Autodesk Inventor part; units mm, degrees
ref_plane "YZ Plane" through (0, 0, 0) normal (1, 0, 0) x (0, 1, 0)
ref_plane "XZ Plane" through (0, 0, 0) normal (0, 1, 0) x (-1, 0, 0)
ref_plane "XY Plane" through (0, 0, 0) normal (0, 0, 1) x (1, 0, 0)
sketch "Эскиз1" plane through (0, 0, 0) normal (0, 1, 0) x (-1, 0, 0)
  arc A0 (13.2517, 5.1196) -> (11.6396, 8.8847) centre (11.8859, 6.7625) ccw
  line L0 (11.6396, 8.8847) -> (3.5765, 5.9707)
  line L1 (3.5765, 5.9707) -> (2.1921, 14.0362)
  arc A1 (2.1921, 14.0362) -> (-1.8746, 14.5225) centre (0.0865, 13.6747) ccw
  line L2 (-1.8746, 14.5225) -> (-3.3825, 6.0827)
  line L3 (-3.3825, 6.0827) -> (-11.0596, 8.9165)
  arc A2 (-11.0596, 8.9165) -> (-13.5142, 5.6378) centre (-11.7994, 6.9122) ccw
  line L4 (-13.5142, 5.6378) -> (-6.959, 0.112)
  line L5 (-6.959, 0.112) -> (-13.2517, -5.1196)
  arc A3 (-13.2517, -5.1196) -> (-11.6396, -8.8847) centre (-11.8859, -6.7625) ccw
  line L6 (-11.6396, -8.8847) -> (-3.5765, -5.9707)
  line L7 (-3.5765, -5.9707) -> (-2.1921, -14.0362)
  arc A4 (-2.1921, -14.0362) -> (1.8746, -14.5225) centre (-0.0865, -13.6747) ccw
  line L8 (1.8746, -14.5225) -> (3.3825, -6.0827)
  line L9 (3.3825, -6.0827) -> (11.0596, -8.9165)
  arc A5 (11.0596, -8.9165) -> (13.5142, -5.6378) centre (11.7994, -6.9122) ccw
  line L10 (13.5142, -5.6378) -> (6.959, -0.112)
  line L11 (6.959, -0.112) -> (13.2517, 5.1196)
  circle A6 centre (6.6709, 3.7954) radius 1
  circle A7 centre (11.8859, 6.7625) radius 1
  circle A8 centre (9.2109, -5.3958) radius 1
  circle A9 centre (-0.0485, -7.6748) radius 1
  circle A10 centre (-0.0865, -13.6747) radius 1
  circle A11 centre (-9.2784, -5.2789) radius 1
  circle A12 centre (-6.6223, 3.8794) radius 1
  circle A13 centre (-11.7994, 6.9122) radius 1
  circle A14 centre (0.0675, 10.6748) radius 1
  circle A15 centre (0, 0) radius 4.75
  circle A16 centre (0.0865, 13.6747) radius 1
  circle A17 centre (0.0485, 7.6748) radius 1
  circle A18 centre (-9.2109, 5.3958) radius 1
  circle A19 centre (-11.8859, -6.7625) radius 1
  circle A20 centre (-6.6709, -3.7954) radius 1
  circle A21 centre (-0.0675, -10.6748) radius 1
  circle A22 centre (11.7994, -6.9122) radius 1
  circle A23 centre (6.6223, -3.8794) radius 1
  circle A24 centre (9.2784, 5.2789) radius 1
  circle A25 centre (0, 0) radius 1.875
  circle A26 centre (0, 0) radius 20
  circle A27 centre (0, 0) radius 17.5
  point P0 (0, 0)
  dimension "d0" = 40
  dimension "d1" = 35
extrude "Выдавливание1" add sketch "Эскиз1" along normal blind 2 contours L11 L10 A5 L9 L8 A4 L7 L6 A3 L5 L4 A2 L3 L2 A1 L1 L0 A0 | A26 | A27
sketch "Эскиз2" plane through (0, 2, 0) normal (0, 1, 0) x (1, 0, 0)
  arc A0 (13.2517, 5.1196) -> (11.6396, 8.8847) centre (11.8859, 6.7625) ccw
  line L0 (11.6396, 8.8847) -> (3.5765, 5.9707)
  line L1 (3.5765, 5.9707) -> (2.1921, 14.0362)
  arc A1 (2.1921, 14.0362) -> (-1.8746, 14.5225) centre (0.0865, 13.6747) ccw
  line L2 (-1.8746, 14.5225) -> (-3.3825, 6.0827)
  line L3 (-3.3825, 6.0827) -> (-11.0596, 8.9165)
  arc A2 (-11.0596, 8.9165) -> (-13.5142, 5.6378) centre (-11.7994, 6.9122) ccw
  line L4 (-13.5142, 5.6378) -> (-6.959, 0.112)
  line L5 (-6.959, 0.112) -> (-13.2517, -5.1196)
  arc A3 (-13.2517, -5.1196) -> (-11.6396, -8.8847) centre (-11.8859, -6.7625) ccw
  line L6 (-11.6396, -8.8847) -> (-3.5765, -5.9707)
  line L7 (-3.5765, -5.9707) -> (-2.1921, -14.0362)
  arc A4 (-2.1921, -14.0362) -> (1.8746, -14.5225) centre (-0.0865, -13.6747) ccw
  line L8 (1.8746, -14.5225) -> (3.3825, -6.0827)
  line L9 (3.3825, -6.0827) -> (11.0596, -8.9165)
  arc A5 (11.0596, -8.9165) -> (13.5142, -5.6378) centre (11.7994, -6.9122) ccw
  line L10 (13.5142, -5.6378) -> (6.959, -0.112)
  line L11 (6.959, -0.112) -> (13.2517, 5.1196)
  circle A6 centre (6.6709, 3.7954) radius 1
  circle A7 centre (11.8859, 6.7625) radius 1
  circle A8 centre (9.2109, -5.3958) radius 1
  circle A9 centre (-0.0485, -7.6748) radius 1
  circle A10 centre (-0.0865, -13.6747) radius 1
  circle A11 centre (-9.2784, -5.2789) radius 1
  circle A12 centre (-6.6223, 3.8794) radius 1
  circle A13 centre (-11.7994, 6.9122) radius 1
  circle A14 centre (0.0675, 10.6748) radius 1
  circle A15 centre (0, 0) radius 4.75
  circle A16 centre (0.0865, 13.6747) radius 1
  circle A17 centre (0.0485, 7.6748) radius 1
  circle A18 centre (-9.2109, 5.3958) radius 1
  circle A19 centre (-11.8859, -6.7625) radius 1
  circle A20 centre (-6.6709, -3.7954) radius 1
  circle A21 centre (-0.0675, -10.6748) radius 1
  circle A22 centre (11.7994, -6.9122) radius 1
  circle A23 centre (6.6223, -3.8794) radius 1
  circle A24 centre (9.2784, 5.2789) radius 1
  circle A25 centre (0, 0) radius 1.875
  circle A26 centre (0, 0) radius 20
  circle A27 centre (0, 0) radius 17.5
  point P0 (0, 0)
  dimension "d4" = 40
  dimension "d5" = 35
extrude "Выдавливание2" add sketch "Эскиз2" along normal blind 6 contours A26
sketch "Эскиз3" plane through (0, 0, 0) normal (0, -1, 0) x (1, 0, 0)
  circle A0 centre (0, 0) radius 20
  line L0 (15.264, 12.9232) -> (15.264, -12.9232)
  line L1 (15.264, 12.9232) -> (35.264, 12.9232)
  line L2 (35.264, 12.9232) -> (35.264, -12.9232)
  line L3 (35.264, -12.9232) -> (15.264, -12.9232)
  line L4 (15.264, -12.9232) -> (15.264, 12.9232)
  dimension "d8" = 20
extrude "Выдавливание3" add sketch "Эскиз3" against normal blind 3 contours A0 L1 L2 L3
sketch "Эскиз4" plane through (0, 0, 0) normal (0, -1, 0) x (1, 0, 0)
  line L0 (35.264, 12.9232) -> (35.264, -12.9232)
  line L1 (35.264, 0) -> (30.264, 0)
  circle A0 centre (30.264, 0) radius 2
  point P0 (0, 0)
  dimension "d17" = 5
  dimension "d18" = 4
extrude "Выдавливание4" cut sketch "Эскиз4" against normal blind 4
sketch "Эскиз5" plane through (0, 0, 0) normal (0, -1, 0) x (1, 0, 0)
  circle A0 centre (0, 0) radius 9
  dimension "d24" = 18
extrude "Выдавливание5" add sketch "Эскиз5" along normal blind 6
sketch "Эскиз6" plane through (0, 2, 0) normal (0, 1, 0) x (1, 0, 0)
  circle A0 centre (0, 0) radius 3
  dimension "d27" = 6
extrude "Выдавливание6" cut sketch "Эскиз6" against normal through all
sketch "Эскиз7" plane through (0, 2, 0) normal (0, 1, 0) x (1, 0, 0)
  circle A0 centre (0, 0) radius 6
  dimension "d30" = 12
extrude "Выдавливание7" cut sketch "Эскиз7" against normal blind 5
pattern_linear "Прямоуг.массив2" count 3 spacing 8 along (0, 0, -1) of "Выдавливание4" first direction both ways yes
chamfer "Фаска3" distance 11 angle 45 3 edges at (15.264, 1.5, -12.9232) (15.264, 1, 12.9232) (15.264, 2.5, 12.9232)
chamfer "Фаска4" distance 9 angle 45 2 edges at (26.264, 2.5, 12.9232) (26.264, 1.5, -12.9232)
properties part number "000.403 - Рычаг" material "Пластик АБС"
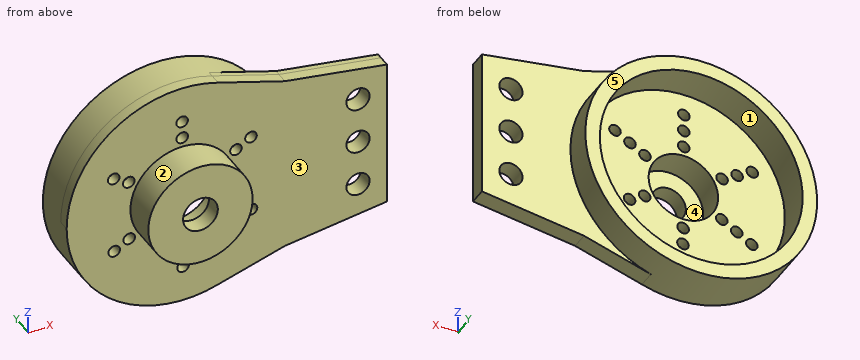
Could you check a few things on this model? Use its own coordinates, in mm. Face numbers are marked on the shaded views. A direction names the side the tool comes from. Give positions to 0.01 mm unless a question says otherwise; leave off trailing zeros. Order: outer loops, then holes, each group sorted by start corner. A loop starts at its lowest first (then second) coordinate and runs counter-clockwise, first axis right, second up.
Q1. If I drill on line 1 along Y through (x, z) = (21.5, 11); line 2 along Y through (x, z) = (-15.5, 0); line 3 along X through (y, z) = (-0.5, 4.5), over which ranges is the centre line in solid material (lowest first)?
Q2. Suppose I cut it at C-C, the plane y = 1. Count the separate pieces of the cut face and the enclosed holes in it, and give its area (3 significant figures).
Q3. Suppose I cut it at B-B, the plane x = 11.5. Write out the boundary of the cut face in (y, z).
Q4. I'm going to push flat-ended pins straight in: P1, Ø1.2, axis at x = -11.8, z = -6.91, coming from the +Y side; P2, Ø1.5, axis at y = -4, z = -7, coming from the -X side; P3, Ø1, axis at x = 3, y = 4.5, coming from the +Z side; P4, Ø2.5, axis at x = -9.28, z = 5.28, coming from the -Y side. Where does each tip first touch, or does it pass through?
Q5. Suppose I cut it at A-A, the plane z = 1. Write out the boundary of the cut face in (x, y), and give its area (3 significant figures).
Q6. Suppose I cut it at D-D, the plane x = -7. Write out the boundary of the cut face in (y, z) (3 decimals), and give its area (3 significant figures).
Q7. We'd pull the mould along X, two halves only. Please class the marked faces 1, 2 and 3: +X half, -X half, draft (parallel to the pull), parting line (faces both ways), or undercut.
Q8. For the marked faces 4 and 5, which set-ups out of +Z, -Z, +X, -X, +Y, -Y let a thin tool reach every point of the face, with its end or its side?
Solution:
1. line 1: y = 0 to 3
1. line 2: y = 0 to 2
1. line 3: x = -7.79 to -3.97, 3.97 to 7.79
2. separate pieces: 1
2. enclosed holes: 22
2. area: 1,560 mm2
3. outline: (0, -17.41) - (3, -17.41) - (3, -16.36) - (8, -16.36) - (8, -13.19) - (2, -13.19) - (2, -7.69) - (0, -7.69) - close; (0, -5.84) - (2, -5.84) - (2, 5.96) - (0, 5.96) - close; (0, 7.87) - (2, 7.87) - (2, 13.19) - (8, 13.19) - (8, 16.36) - (3, 16.36) - (3, 17.41) - (0, 17.41) - close
4. P1: passes through
4. P2: stops at x = -6.48
4. P3: stops at z = 19.84
4. P4: stops at y = 0
5. outline: (-19.97, 0) - (-8.94, 0) - (-8.94, -6) - (-2.83, -6) - (-2.83, -3) - (-5.92, -3) - (-5.92, 2) - (-17.47, 2) - (-17.47, 8) - (-19.97, 8) - close; (2.83, -6) - (8.94, -6) - (8.94, 0) - (28.53, 0) - (28.53, 3) - (19.97, 3) - (19.97, 8) - (17.47, 8) - (17.47, 2) - (5.92, 2) - (5.92, -3) - (2.83, -3) - close; (32, 0) - (35.26, 0) - (35.26, 3) - (32, 3) - close
5. area: 177 mm2
6. outline: (-6, -5.657) - (0, -5.657) - (0, -18.735) - (8, -18.735) - (8, -16.039) - (2, -16.039) - (2, -4.805) - (0, -4.805) - (0, -2.953) - (2, -2.953) - (2, 2.851) - (0, 2.851) - (0, 4.74) - (2, 4.74) - (2, 16.039) - (8, 16.039) - (8, 18.735) - (0, 18.735) - (0, 5.657) - (-6, 5.657) - close
6. area: 168 mm2
7. face 1: undercut
7. face 2: parting line
7. face 3: draft
8. face 4: +Y
8. face 5: +Z, -Z, +X, -X, +Y
